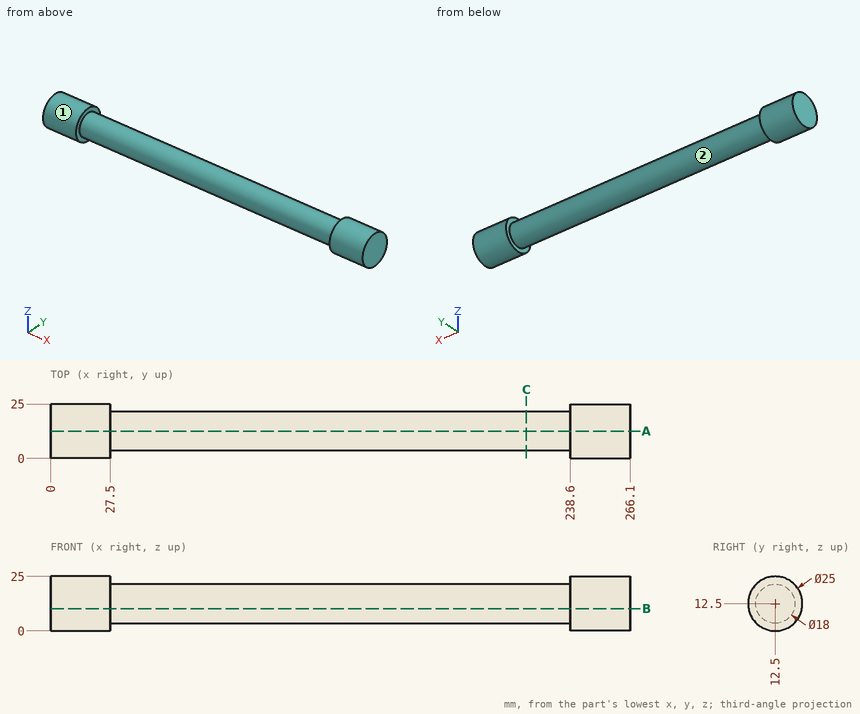
Design review of the part shown in the three views and the two pictorial views. Dimensions are in mm from the part's minimum x, y and z. A direction names the side the tool comes from. Give positions to 0.01 mm unless a question says otherwise; leave off trailing zeros. Write each loop counter-clockwise with the first axis right and the second up, starting at its lowest first coordinate (ties: lowest second). Pieces come first, ordered by that corner, then holes. Notation, with made-up numbers: M -14,42.5 L 2,42.5 A18 cw 2,72.5 Z; hole C 41.5,29.25 d9. An arc over 180 degrees is marked long. One line per item, written item: value.
1) Take a section at C-C, the plane x = 218.5. Write out the cut boundary in (y, z).
Results are:
outline: C 12.5,12.5 d18
2) Take a section at A-A, the plane y = 12.5. Write out the cut boundary in (x, z), then the cut area to 3 significant figures.
Results are:
outline: M 0,0 L 27.5,0 L 27.5,3.5 L 238.6,3.5 L 238.6,0 L 266.1,0 L 266.1,25 L 238.6,25 L 238.6,21.5 L 27.5,21.5 L 27.5,25 L 0,25 Z
area: 5,170 mm²
3) For line 1 (X direction, y = 23, z = 16.25); line 2 (Z direction, x = 192.5, y = 15); line 3 (Z direction, x = 53.5, y = 13), list the stretches that pass through material, from the lowest coordinate up. Write a range as from..to.
Results are:
line 1: x = 0..27.5, 238.6..266.1
line 2: z = 3.85..21.15
line 3: z = 3.51..21.49
4) For P1, Ø6, axis at x = 85.5, y = 5.5, coming from the +Z side; P2, Ø5, axis at x = 67, y = 11.5, coming from the -Z side; P3, Ø3, axis at y = 11.5, z = 12, coming from the -X side; P4, Ø10, axis at x = 129, z = 18.5, coming from the +Y side, all flat-tipped, find the tip position at first contact; note any pin that passes through.
Results are:
P1: stops at z = 20.56
P2: stops at z = 3.5
P3: stops at x = 0
P4: stops at y = 21.44
5) Take a section at B-B, the plane z = 10.25. Write out the cut boundary in (x, y).
Results are:
outline: M 0,0.2 L 27.5,0.2 L 27.5,3.79 L 238.6,3.79 L 238.6,0.2 L 266.1,0.2 L 266.1,24.8 L 238.6,24.8 L 238.6,21.21 L 27.5,21.21 L 27.5,24.8 L 0,24.8 Z
6) For the marked faces 1 and 2, list the 3-axis set-ups (+Z, -Z, +X, -X, +Y, -Y) from which the entire face can be reached by the end or side of a thin tool; tool diameter is ignored.
Results are:
face 1: +X, -X
face 2: none
